Geometry check sheet. Reference: the model listing, model coordinates, mm. Face numbers are marked on the shaded views. A direction names the side the tool comes from. Give positions to 0.01 mm unless a question says otherwise; leave off trailing zeros. Write each loop counter-clockwise with the first axis right and the second up, starting at its lowest first coordinate (ties: lowest second). Pieces come first, ordered by that corner, then holes. Notation, with made-up numbers: (34.5, 55.5) - (78.5, 55.5) arc R34 cw to (78.5, 89.5) - close; hole circle Ø7 at (61, 75). An arc over 180 degrees is marked (long way). Write item = value, one per line. Start each with the question number.
(1) Draft check along Z on the marked faces 1, 2, 3 and 4. Enter one of: pulls with the +Z half, pulls with the -Z half, needs draft (parallel to the pull), parting line crosses it, or undercut.
(2) Section check C-C, the plane y = -16. Enter the section's corners in (x, z).
(3) Depth check by flat-ended pin: pin 1 Ø5 at (y, z) = (-16, 2.5) entering from -X (3 decimals); pin 2 Ø1 at (x, z) = (16, 2) entering from +Y; pin 3 Ø6 at (y, z) = (0, 11.5) entering from -X. Enter the tip coordinate at first touch or a pass-through.
(4) Thickness scan on L1, parallel to Y at x = -14.95, z = 11.5; L2, parallel to Y at x = 0, z = 12; L3, parallel to Z at x = -14.35, y = 0. Record the ranges inside material, lowest first.
(5) Access from +Z, -Z, +X, -X, +Y, -Y to the whole of each face (thin tool, end or side, straight path). Record for the marked faces 5 and 6.
(6) Section check D-D, the plane y = -8.25. Enter the section's corners in (x, z).
(7) Section check A-A, the plane x = 0. Enter the section's corners in (y, z), plus the area to 3 significant figures.
(8) Section check B-B, the plane z = 9.25. Give the number of separate pieces and of enclosed holes in the cut face, plus the area to 3 significant figures.
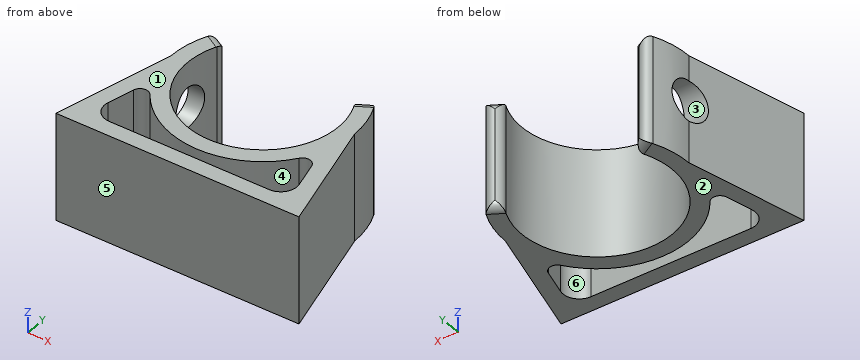
```python
from build123d import *

# Parameters (mm, degrees)
BOSS_EXTRUDE1_DEPTH = 20
BOSS_EXTRUDE2_START = -20
BOSS_EXTRUDE2_DEPTH = 20
FILLET1_R           = 1.5
FILLET2_R           = 1.5
SKETCH3_R           = 3.75
CUT_EXTRUDE1_DEPTH  = 20


with BuildPart() as part:
    # Sketch1 → Boss-Extrude1 (new body)
    with BuildSketch(Plane.XY):
        with BuildLine():
            Line((12.14432037, 6.965305646), (14.746674735, 8.457871142))
            ThreePointArc((14.746674735, 8.457871142), (-0.048606097, -16.999930513), (-14.698068638, 8.542059371))
            Line((-14.698068638, 8.542059371), (-12.10429182, 7.034637129))
            ThreePointArc((-12.10429182, 7.034637129), (-0.04002855, -13.999942775), (12.14432037, 6.965305646))
        make_face()
    extrude(amount=BOSS_EXTRUDE1_DEPTH)

    # Sketch2 → Boss-Extrude2 (add)
    with BuildSketch(Plane.XY.offset(20).offset(BOSS_EXTRUDE2_START)):
        with BuildLine():
            Line((-17, 0), (-22.5, -22))
            Line((-22.5, -22), (22.5, -22))
            Line((22.5, -22), (17, 0))
            ThreePointArc((17, 0), (16.645771335, -3.452288612), (15.597847452, -6.760706684))
            Line((15.597847452, -6.760706684), (17.725769062, -15.272393125))
            ThreePointArc((17.725769062, -15.272393125), (17.179957876, -17.846236628), (14.815341562, -19))
            Line((14.815341562, -19), (-14.815341562, -19))
            ThreePointArc((-14.815341562, -19), (-17.179957876, -17.846236628), (-17.725769062, -15.272393125))
            Line((-17.725769062, -15.272393125), (-15.597847452, -6.760706684))
            ThreePointArc((-15.597847452, -6.760706684), (-16.645771335, -3.452288612), (-17, 0))
        make_face()
    extrude(amount=BOSS_EXTRUDE2_DEPTH)

    # Fillet1
    fillet1_edges = [part.edges().sort_by_distance(p)[0] for p in [
        (-15.597847452, -6.760706684, 10),
        (15.597847452, -6.760706684, 10),
    ]]
    fillet(fillet1_edges, radius=FILLET1_R)

    # Fillet2
    fillet2_edges = [part.edges().sort_by_distance(p)[0] for p in [
        (13.445497553, 7.711588394, 20),
        (13.445497553, 7.711588394, 0),
        (-13.401180229, 7.78834825, 0),
        (12.14432037, 6.965305646, 10),
        (14.746674735, 8.457871142, 10),
        (-14.698068638, 8.542059371, 10),
        (-12.10429182, 7.034637129, 10),
        (-13.401180229, 7.78834825, 20),
    ]]
    fillet(fillet2_edges, radius=FILLET2_R - 0.0001)  # a hair under: the kernel refuses the full size

    # Sketch3 → Cut-Extrude1 (cut)
    with BuildSketch(Plane(origin=(0, 0, 0), x_dir=(0, 0, -1), z_dir=(1, 0, 0))):
        with Locations((-11.5, 0)):
            Circle(SKETCH3_R)
    extrude(amount=-CUT_EXTRUDE1_DEPTH, mode=Mode.SUBTRACT)


solid = part.part
```
Model answer:
q1.face_1 = pulls with the +Z half
q1.face_2 = pulls with the -Z half
q1.face_3 = undercut
q1.face_4 = needs draft
q2.outline = (-21, 0) - (-17.82, 0) - (-17.82, 20) - (-21, 20) - close; (-5.74, 0) - (5.74, 0) - (5.74, 20) - (-5.74, 20) - close; (17.82, 0) - (21, 0) - (21, 20) - (17.82, 20) - close
q3.pin_1 = -21.625
q3.pin_2 = 6.98
q3.pin_3 = 13.67
q4.L1 = -22 to -19, -9.26 to -3.75, 3.75 to 7.69
q4.L2 = -22 to -19, -17 to -14
q4.L3 = 0 to 7.75, 15.25 to 20
q5.face_5 = +Z, -Z, +X, -X, -Y
q5.face_6 = +Z, -Z
q6.outline = (-19.06, 0) - (-11.31, 0) - (-11.31, 20) - (-19.06, 20) - close; (11.31, 0) - (19.06, 0) - (19.06, 20) - (11.31, 20) - close
q7.outline = (-22, 0) - (-19, 0) - (-19, 20) - (-22, 20) - close; (-17, 0) - (-14, 0) - (-14, 20) - (-17, 20) - close
q7.area = 120 mm²
q8.separate_pieces = 2
q8.enclosed_holes = 1
q8.area = 412 mm²
